Read the model definition and answer for the solid it produces. Units are mm, in the model's axes. Coordinates: 2 decimals unless noted, no trailing zeros. Write each loop counter-clockwise with the first axis right and the second up, starting at its lowest first coordinate (ties: lowest second). Pieces come first, ordered by that corner, then holes. Notation, with made-up numbers: M 54,29 L 100,29 A28 cw 100,68 Z; hole C 87,78 d4. An arc over 180 degrees is marked long. Use a Markdown table: item, result. Add a question column.
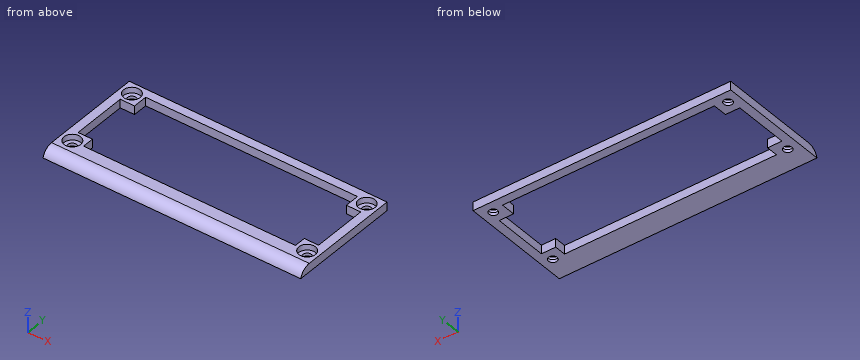
Autodesk Inventor part; units mm, degrees
ref_plane "YZ Plane" through (0, 0, 0) normal (1, 0, 0) x (0, 1, 0)
ref_plane "XZ Plane" through (0, 0, 0) normal (0, 1, 0) x (-1, 0, 0)
ref_plane "XY Plane" through (0, 0, 0) normal (0, 0, 1) x (1, 0, 0)
sketch "スケッチ1" plane through (0, 0, 0) normal (0, 0, 1) x (1, 0, 0)
  line L0 (-45, 3.5) -> (45, 3.5)
  line L1 (45, 3.5) -> (45, -3.5)
  line L2 (45, -3.5) -> (-45, -3.5)
  line L3 (-45, -3.5) -> (-45, 3.5)
  line L4 (-45, 3.5) -> (45, -3.5) construction
  line L5 (45, 3.5) -> (-45, -3.5) construction
  point P0 (0, 0)
  dimension "d0" = 90
  dimension "d1" = 7
extrude "押し出し1" add sketch "スケッチ1" along normal blind 3
sketch "スケッチ2" plane through (0, 0, 3) normal (0, 0, 1) x (1, 0, 0)
  circle A0 centre (-41, -0.4) radius 2.9
  circle A1 centre (41, -0.4) radius 2.9
  line L0 (45, 3.5) -> (-45, 3.5)
  line L1 (45, -3.5) -> (45, 3.5)
  point P0 (0, 0)
  dimension "d4" = 5.8
  dimension "d5" = 5.8
  dimension "d7" = 3.9
  dimension "d8" = 3.9
  dimension "d9" = 82
  dimension "d10" = 4
extrude "押し出し2" cut sketch "スケッチ2" against normal blind 2
sketch "スケッチ3" plane through (0, 0, 0) normal (0, 0, -1) x (-1, 0, 0)
  circle A0 centre (41, -0.4) radius 1.5
  circle A1 centre (-41, -0.4) radius 1.5
  line L0 (45, -3.5) -> (45, 3.5)
  line L1 (-45, 3.5) -> (-45, -3.5)
  line L2 (45, 3.5) -> (-45, 3.5)
  point P0 (0, 0)
  dimension "d13" = 3
  dimension "d14" = 3
  dimension "d15" = 4
  dimension "d16" = 4
  dimension "d17" = 3.9
  dimension "d18" = 3.9
extrude "押し出し3" cut sketch "スケッチ3" against normal blind 2
sketch "スケッチ4" plane through (-45, -3.5, 0) normal (0, -1, 0) x (1, 0, 0)
  line L0 (0, 0) -> (90, 0)
  line L1 (90, 0) -> (90, 3)
  line L2 (90, 3) -> (0, 3)
  line L3 (0, 3) -> (0, 0)
  point P0 (45, 0)
extrude "押し出し4" add sketch "スケッチ4" along normal blind 5
fillet "フィレット1" radius 4 1 edges at (0, -8.5, 3)
sketch "スケッチ6" plane through (0, 0, 0) normal (0, 0, -1) x (-1, 0, 0)
  line L0 (37, -0.5) -> (-37, -0.5)
  line L1 (-37, -0.5) -> (-37, 3.5)
  line L2 (-37, 3.5) -> (37, 3.5)
  line L3 (37, 3.5) -> (37, -0.5)
  line L4 (45, -8.5) -> (45, 3.5)
  line L5 (45, 3.5) -> (-45, 3.5)
  point P0 (0, 0)
  dimension "d24" = 74
  dimension "d25" = 8
  dimension "d26" = 0
  dimension "d27" = 4
extrude "押し出し5" cut sketch "スケッチ6" against normal blind 10
sketch "スケッチ7" plane through (45, 3.5, 3) normal (0, 1, 0) x (1, 0, 0)
  line L0 (0, 3) -> (-3, 3)
  line L1 (-3, 3) -> (-3, 0)
  line L2 (-3, 0) -> (0, 0)
  line L3 (0, 0) -> (0, 3)
  line L4 (-90, 0) -> (-87, 0)
  line L5 (-87, 0) -> (-87, 3)
  line L6 (-87, 3) -> (-90, 3)
  line L7 (-90, 3) -> (-90, 0)
  point P0 (-45, 3)
  dimension "d30" = 3
  dimension "d31" = 3
  dimension "d32" = 3
  dimension "d33" = 3
extrude "押し出し6" add sketch "スケッチ7" along normal blind 27.1
sketch "スケッチ8" plane through (-42, 3.5, 3) normal (1, 0, 0) x (0, 0, -1)
  line L0 (0, 27.1) -> (3, 27.1)
  line L1 (3, 27.1) -> (3, 24.1)
  line L2 (3, 24.1) -> (0, 24.1)
  line L3 (0, 24.1) -> (0, 27.1)
  point P0 (3, -3.5)
  dimension "d36" = 3
  dimension "d37" = 3
extrude "押し出し7" add sketch "スケッチ8" along normal blind 86
sketch "スケッチ9" plane through (0, 0, 3) normal (0, 0, 1) x (1, 0, 0)
  line L0 (-45, 30.6) -> (-37, 30.6)
  line L1 (-37, 30.6) -> (-37, 22.6)
  line L2 (-37, 22.6) -> (-45, 22.6)
  line L3 (-45, 22.6) -> (-45, 30.6)
  line L4 (45, 30.6) -> (37, 30.6)
  line L5 (37, 30.6) -> (37, 22.6)
  line L6 (37, 22.6) -> (45, 22.6)
  line L7 (45, 22.6) -> (45, 30.6)
  point P0 (0, 0)
  dimension "d40" = 8
  dimension "d41" = 8
  dimension "d42" = 8
  dimension "d43" = 8
extrude "押し出し8" add sketch "スケッチ9" against normal blind 3
sketch "スケッチ10" plane through (0, 0, 3) normal (0, 0, 1) x (1, 0, 0)
  circle A0 centre (-41, 26.6) radius 1.5
  circle A1 centre (41, 26.6) radius 1.5
  line L0 (-45, 30.6) -> (45, 30.6)
  line L1 (-45, -4.627) -> (-45, 30.6)
  line L2 (45, 30.6) -> (45, -4.627)
  point P0 (0, 0)
  dimension "d46" = 4
  dimension "d47" = 4
  dimension "d50" = 3
  dimension "d51" = 3
  dimension "d52" = 4
  dimension "d53" = 4
extrude "押し出し9" cut sketch "スケッチ10" against normal blind 3
sketch "スケッチ11" plane through (0, 0, 3) normal (0, 0, 1) x (1, 0, 0)
  circle A0 centre (-41, 26.6) radius 1.5
  circle A1 centre (-41, 26.6) radius 2.9
  circle A2 centre (41, 26.6) radius 2.9
  line L0 (-45, 30.6) -> (45, 30.6)
  line L1 (45, 30.6) -> (45, -4.627)
  point P0 (0, 0)
  dimension "d56" = 5.8
  dimension "d57" = 5.8
  dimension "d58" = 4
  dimension "d60" = 4
extrude "押し出し10" cut sketch "スケッチ11" against normal blind 2
properties part number "LineTraceCoverFlont"
Item 1: Consider probe 1 along Y at (x, z) = (-41, 0.2); probe 2 along Y at (x, z) = (-41, 1.75); probe 3 along X at (y, z) = (10, 0.7). Determine where each line is inside the solid, lowest interval first.
Item 2: Each of these flat-tipped pins is pushed along its axis until it touches: pin 1 (2.5 mm diameter, centred on x = -41, y = -0.4, fed in from -Z); pin 2 (3 mm diameter, centred on x = -40, y = -0.5, fed in from +Z); pin 3 (1 mm diameter, centred on x = -29.5, z = 2.5, fed in from -Y); pin 4 (1.5 mm diameter, centred on x = -1, z = 2, fed in from -Y). Where does it stop, or does it pass through?
Item 3: Find section D-D on x = 41. Give the vertices of the cut face in (y, z), then the cut area to 3 significant figures.
Item 4: Find section A-A on y = 26.6. Give the vertices of the cut face in (x, z).
Item 5: Find section B-B on x = -11. Give the vertices of the cut face in (y, z), then the cut area to 3 significant figures.
Item 6: Find section C-C on y = 14.5. Give the vertices of the cut face in (x, z), then the cut area to 3 significant figures.
Geometry says:
| question | item | result |
|---|---|---|
| 1 | probe 1 | y = -8.44 to -1.9, 1.1 to 3.5, 22.6 to 25.1, 28.1 to 30.6 |
| 1 | probe 2 | y = -7.53 to -3.3, 2.5 to 3.5, 22.6 to 23.7, 29.5 to 30.6 |
| 1 | probe 3 | x = -45 to -42, 42 to 45 |
| 2 | pin 1 | passes through |
| 2 | pin 2 | stops at z = 1 |
| 2 | pin 3 | stops at y = -7.27 |
| 2 | pin 4 | stops at y = -7.93 |
| 3 | outline | M -8.5,0 L -1.9,0 L -1.9,1 L -3.3,1 L -3.3,3 L -4.63,3 A4 ccw Z; M 1.1,0 L 3.5,0 L 3.5,3 L 2.5,3 L 2.5,1 L 1.1,1 Z; M 22.6,0 L 25.1,0 L 25.1,1 L 23.7,1 L 23.7,3 L 22.6,3 Z; M 28.1,0 L 30.6,0 L 30.6,3 L 29.5,3 L 29.5,1 L 28.1,1 Z |
| 3 | area | 27.8 mm2 |
| 4 | outline | M -45,0 L -42.5,0 L -42.5,1 L -43.9,1 L -43.9,3 L -45,3 Z; M -39.5,0 L -37,0 L -37,3 L -38.1,3 L -38.1,1 L -39.5,1 Z; M 37,0 L 39.5,0 L 39.5,1 L 38.1,1 L 38.1,3 L 37,3 Z; M 42.5,0 L 45,0 L 45,3 L 43.9,3 L 43.9,1 L 42.5,1 Z |
| 5 | outline | M -8.5,0 L -0.5,0 L -0.5,3 L -4.63,3 A4 ccw Z; M 27.6,0 L 30.6,0 L 30.6,3 L 27.6,3 Z |
| 5 | area | 30.0 mm2 |
| 6 | outline | M -45,0 L -42,0 L -42,3 L -45,3 Z; M 42,0 L 45,0 L 45,3 L 42,3 Z |
| 6 | area | 18.0 mm2 |
